from build123d import *

# Parameters (mm, degrees)
ESBO_O1_R                = 20
RESSALTO_EXTRUS_O1_DEPTH = 8
ESBO_O2_R                = 12.7
RESSALTO_EXTRUS_O2_DEPTH = 15
CHANFRO1_SIZE            = 1
ESBO_O3_R                = 8
CORTE_EXTRUS_O1_DEPTH    = 15
ESBO_O4_R                = 6
CORTE_EXTRUS_O2_DEPTH    = 37.455452267
CHANFRO2_SIZE            = 1


with BuildPart() as part:
    # Esboço1 → Ressalto-extrusão1 (new body)
    with BuildSketch(Plane.XY):
        Circle(ESBO_O1_R)
    extrude(amount=RESSALTO_EXTRUS_O1_DEPTH)

    # Esboço2 → Ressalto-extrusão2 (add)
    with BuildSketch(Plane.XY.offset(8)):
        Circle(ESBO_O2_R)
    extrude(amount=RESSALTO_EXTRUS_O2_DEPTH)

    # Chanfro1
    chanfro1_edges = [part.edges().sort_by_distance(p)[0] for p in [
        (-12.7, 0, 23),
    ]]
    chamfer(chanfro1_edges, length=CHANFRO1_SIZE)

    # Esboço3 → Corte-extrusão1 (cut)
    with BuildSketch(Plane.XY.offset(23)):
        Circle(ESBO_O3_R)
    extrude(amount=-CORTE_EXTRUS_O1_DEPTH, mode=Mode.SUBTRACT)

    # Esboço4 → Corte-extrusão2 (cut, through all)
    with BuildSketch(Plane(origin=(0, 0, 0), x_dir=(-1, 0, 0), z_dir=(0, 0, -1))):
        Circle(ESBO_O4_R)
    extrude(amount=-CORTE_EXTRUS_O2_DEPTH, mode=Mode.SUBTRACT)

    # Chanfro2
    chanfro2_edges = [part.edges().sort_by_distance(p)[0] for p in [
        (-20, 0, 0),
        (-20, 0, 8),
    ]]
    chamfer(chanfro2_edges, length=CHANFRO2_SIZE)


solid = part.part
Source: CAD feature listing. Evaluate the final solid. Frame: model axes, mm. A direction names the side the tool comes from. Coordinates: 2 decimals unless noted, no trailing zeros. Loops run counter-clockwise (first coordinate to the right, second up) from the corner with the lowest first, then second, coordinate; pieces in that order, holes last. Notation, with made-up numbers: (66, -35) - (117, -35) arc R20 ccw to (117, -3) - close; hole circle Ø4 at (-30.75, 75.5). An arc over 180 degrees is marked (long way). One line per item, written item: value. Start each with the question number.
1. Section A-A (y = 0). Return the cut outline in (x, z), and give its area (3 significant figures).
2. Mould query, pull axis X, two halves, no side actions, for faces 3 (the cylindrical face through (-2.75, -12.4, 14.9)), 4 (the flat face through (-4.5, 4.5, 0)), 5 (the cylindrical face through (-1.73, -7.81, 15.6)). Classes: pulls with the +X half, pulls with the -X half, needs draft (parallel to the pull), parting line crosses it, or undercut.
3. Contact query for flat-ended pins moving along their axis: P1, Ø6, axis at x = 7, z = 6, coming from the -Y side; P2, Ø10, axis at x = -7, z = 19, coming from the -Y side; P3, Ø5, axis at x = 0.5, z = 16.5, coming from the -Y side. Output: stop coordinate, or through.
4. Section C-C (z = 16.25). Return the cut outline in (x, y), and give its area (3 significant figures).
5. Ray query, L1, parallel to Z at x = -12.5, y = 7.5; L2, parallel to Y at x = 6, z = 18; L3, parallel to X at y = -2, z = 9. Return the intervals inside material, ascending.
6. Set-up query: faces 1 (the flat face through (12.4, -4, 8)), 2 (the cylindrical face through (-4.336, -19.524, 3.958)). Return all of +Z, -Z, +X, -X, +Y, -Y with unobstructed straight access to the full face (end or side cutting, diameter ignored); none if empty.
Verdict:
1. outline: (-20, 1) - (-19, 0) - (-6, 0) - (-6, 8) - (-8, 8) - (-8, 23) - (-11.7, 23) - (-12.7, 22) - (-12.7, 8) - (-19, 8) - (-20, 7) - close; (6, 0) - (19, 0) - (20, 1) - (20, 7) - (19, 8) - (12.7, 8) - (12.7, 22) - (11.7, 23) - (8, 23) - (8, 8) - (6, 8) - close
1. area: 362 mm2
2. face 3: parting line crosses it
2. face 4: needs draft
2. face 5: undercut
3. P1: stops at y = -19.6
3. P2: stops at y = -12.54
3. P3: stops at y = -12.7
4. outline: circle Ø25.4 at (0, 0); hole circle Ø16 at (0, 0)
4. area: 306 mm2
5. L1: z = 0 to 8
5. L2: y = -11.19 to -5.29, 5.29 to 11.19
5. L3: x = -12.54 to -7.75, 7.75 to 12.54
6. face 1: +Z
6. face 2: +Z, -Z
